Here's how the part is built. I have some questions about the finished solid (model axes, mm). Face numbers are marked on the shaded views. A direction names the side the tool comes from. Round coordinates to 2 decimals unless told otherwise and drop trailing zeros. Order: outer loops, then holes, each group sorted by start corner. A loop starts at its lowest first (then second) coordinate and runs counter-clockwise, first axis right, second up. Notation, with made-up numbers: (32.5, -21.75) -> (81.5, -21.75) arc R23 cw to (81.5, -3.75) -> close; hole circle Ø7 at (-1.5, -12.75). An arc over 180 degrees is marked (long way). Use a Markdown table: item, result. Add a question column.
(1) I'm going to push flat-ended pins straight in: P1, Ø1, axis at x = 4, y = -6, coming from the -Z side; P2, Ø3, axis at y = -0.5, z = 3, coming from the -X side; P3, Ø5, axis at x = -12, z = 2.5, coming from the +Y side. Where does each tip first touch, or does it pass through?
(2) I want a section at C-C, the plane x = 4.5. Please give me the cut outline in (y, z).
(3) I want a section at D-D, the plane z = -5.75. Please give me the cut outline in (x, y), then the cut area to 3 significant figures.
(4) I want a section at B-B, the plane y = 18.5. Please give me the cut outline in (x, z), then the cut area to 3 significant figures.
(5) If I drill on probe 1 along X at (y, z) = (21, 0.25); probe 2 along X at (y, z) = (9, 1.75); probe 3 along Z at (x, y) = (7.5, -4.5), over which ranges is the centre line in solid material (lowest first)?
(6) Thinking about a two-plate mould opening in Y: for the marked faces 1, 2, 3 and 4, which applies, pulls with the +Y half, pulls with the -Y half, needs draft (parallel to the pull), parting line crosses it, or undercut?
(7) On a 3-axis mill with a long thin cutter (end or side, diameter ignored), from which of +Z, -Z, +X, -X, +Y, -Y can I reach the whole of each face in a straight line? I mean the marked faces 5 and 6. Say none if no direction works.
(8) I want a section at A-A, the plane z = -2.5. Please give me the cut outline in (x, y).
from build123d import *

# Parameters (mm, degrees)
SKETCH1_R           = 10.16
SKETCH1_R_2         = 6.35
REVOLVE1_ANGLE      = 90
SKETCH2_R           = 10.16
SKETCH2_R_2         = 8.001
BOSS_EXTRUDE1_DEPTH = 12.7
SKETCH3_R           = 10.16
SKETCH3_R_2         = 8.001
BOSS_EXTRUDE2_DEPTH = 12.7


with BuildPart() as part:
    # Sketch1 → Revolve1 (revolve)
    with BuildSketch(Plane(origin=(0, 0, 0), x_dir=(0, 0, -1), z_dir=(1, 0, 0))):
        Circle(SKETCH1_R)
        Circle(SKETCH1_R_2, mode=Mode.SUBTRACT)
    revolve(axis=Axis((0, 12.286198988, 1000.032631209), (0, 0, -1)), revolution_arc=REVOLVE1_ANGLE)

    # Sketch2 → Boss-Extrude1 (add)
    with BuildSketch(Plane(origin=(0, 12.286198988, 0), x_dir=(1, 0, 0), z_dir=(0, 1, 0))):
        with Locations(Location((-12.286198988, 0, 0), (0, 0, 180))):
            Circle(SKETCH2_R)
        with Locations(Location((-12.286198988, 0, 0), (0, 0, 180))):
            Circle(SKETCH2_R_2, mode=Mode.SUBTRACT)
    extrude(amount=BOSS_EXTRUDE1_DEPTH)

    # Sketch3 → Boss-Extrude2 (add)
    with BuildSketch(Plane(origin=(0, 0, 0), x_dir=(0, 0, -1), z_dir=(1, 0, 0))):
        with Locations(Location((0, 0, 0), (0, 0, 270))):
            Circle(SKETCH3_R)
        Circle(SKETCH3_R_2, mode=Mode.SUBTRACT)
    extrude(amount=BOSS_EXTRUDE2_DEPTH)


solid = part.part
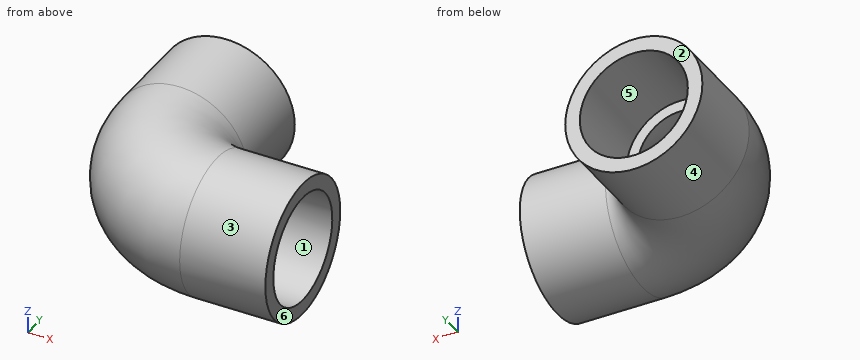
Taken from the geometry:
| question | item | result |
|---|---|---|
| 1 | P1 | stops at z = -8.54 |
| 1 | P2 | stops at x = -18.99 |
| 1 | P3 | stops at y = 2.35 |
| 2 | outline | circle Ø20.32 at (0, 0); hole circle Ø16 at (0, 0) |
| 3 | outline | (-20.66, 12.29) arc R20.66 ccw to (0, -8.38) -> (12.7, -8.38) -> (12.7, -5.56) -> (0, -5.56) -> (0, -2.69) arc R14.98 cw to (-14.98, 12.29) -> (-17.85, 12.29) -> (-17.85, 24.99) -> (-20.66, 24.99) -> close; (-9.59, 12.29) arc R9.59 ccw to (0, 2.69) -> (0, 5.56) -> (12.7, 5.56) -> (12.7, 8.38) -> (0, 8.38) arc R3.91 cw to (-3.91, 12.29) -> (-3.91, 24.99) -> (-6.72, 24.99) -> (-6.72, 12.29) -> close |
| 3 | area | 362 mm2 |
| 4 | outline | circle Ø20.32 at (-12.29, 0); hole circle Ø16 at (-12.29, 0) |
| 4 | area | 123 mm2 |
| 5 | probe 1 | x = -22.44 to -20.28, -4.29 to -2.13 |
| 5 | probe 2 | x = -22.05 to -18.09, -5.24 to 12.7 |
| 5 | probe 3 | z = -9.11 to -6.62, 6.62 to 9.11 |
| 6 | face 1 | undercut |
| 6 | face 2 | pulls with the +Y half |
| 6 | face 3 | parting line crosses it |
| 6 | face 4 | needs draft |
| 7 | face 5 | +Y |
| 7 | face 6 | +Z, -Z, +X, +Y, -Y |
| 8 | outline | (-22.13, 12.29) arc R22.13 ccw to (0, -9.85) -> (12.7, -9.85) -> (12.7, -7.6) -> (0, -7.6) -> (0, -5.84) arc R18.12 cw to (-18.12, 12.29) -> (-19.89, 12.29) -> (-19.89, 24.99) -> (-22.13, 24.99) -> close; (-6.45, 12.29) arc R6.45 ccw to (0, 5.84) -> (0, 7.6) -> (12.7, 7.6) -> (12.7, 9.85) -> (0, 9.85) arc R2.44 cw to (-2.44, 12.29) -> (-2.44, 24.99) -> (-4.69, 24.99) -> (-4.69, 12.29) -> close |
